For this review, take the finished solid that the model builds, in its own axes (mm). Face numbers are marked on the shaded views. A direction names the side the tool comes from. Coordinates: 2 decimals unless noted, no trailing zeros. Write each loop counter-clockwise with the first axis right and the second up, starting at its lowest first coordinate (ties: lowest second). Pieces come first, ordered by that corner, then holes.
1) We need section C-C on y = 40.5. Write out the cut boundary in (x, z).
2) For the marked faces 5, 6 and 7, list the 3-axis set-ups (+Z, -Z, +X, -X, +Y, -Y) from which the entire face can be reached by the end or side of a thin tool; tool diameter is ignored.
3) To check wall thickness, follow line 1 along Z through (x, y) = (1, 63.5); line 2 along X through (y, z) = (192.5, -11.5); line 3 along X through (y, z) = (135.5, -80.5). State the ranges of each line that lie inside material, in increasing order.
4) We need section B-B on x = 18. Write out the cut boundary in (y, z).
5) We need section D-D on x = 0. Write out the cut boundary in (y, z), then the cut area to 3 significant figures.
6) Mouldability with a two-part tool opening along X and no side actions: class the marked faces 1, 2, 3 and 4 as pulls with the +X half, pulls with the -X half, needs draft (parallel to the pull), parting line crosses it, or undercut.
7) We need section A-A on y = 139. Write out the cut boundary in (x, z), then the cut area to 3 significant figures.
8) Insertion check: P1, Ø9.5, axis at y = 68, z = -114, coming from the +X side; P2, Ø16, axis at y = 39.5, z = -13, coming from the -X side; P3, Ø1.5, axis at x = -34.5, z = -61.5, coming from the -Y side. Each pin has a flat end and moves straight along its axis. Give the tip position at first contact, or say it passes through.
from build123d import *

# Parameters (mm, degrees)
SKETCH1_R                = 23.241
FTA_DEPTH                = 127
SKETCH2_W                = 46.482
SKETCH2_H                = 101.6
FTB_DEPTH                = 32.004
FTC_DEPTH                = 127
SKETCH4_W                = 40.64
SKETCH4_H                = 38.1
FTD1_DEPTH               = 127
SKETCH4_5_W              = 40.64
SKETCH4_5_H              = 38.1
FTD2_DEPTH               = 127
SKETCH5_W                = 25.4
SKETCH5_H                = 48.26
FTE_DEPTH                = 127
FTE_2_DEPTH              = 127
SKETCH6_W                = 40.64
SKETCH6_H                = 48.26
SKETCH6_H_2              = 30.48
FILLER_DEPTH             = 127
BOSS_EXTRUDE1_DEPTH      = 16.002
BOSS_EXTRUDE1_DEPTH_BACK = 16.002
SKETCH8_W                = 46.482
SKETCH8_H                = 101.6
CHAMFER1_SIZE            = 7.62
BOSS_EXTRUDE2_DEPTH      = 32.004
CHAMFER2_SIZE            = 25.4
CHAMFER3_SIZE            = 7.62


with BuildPart() as part:
    # Sketch1 → ftA (new body)
    with BuildSketch(Plane.XY):
        Circle(SKETCH1_R)
    extrude(amount=-FTA_DEPTH)


with BuildPart() as body_2:
    # Sketch2 → ftB (new body)
    with BuildSketch(Plane(origin=(0, 0, -127), x_dir=(-1, 0, 0), z_dir=(0, 0, -1))):
        with Locations((0, 50.8)):
            Rectangle(SKETCH2_W, SKETCH2_H)
    extrude(amount=-FTB_DEPTH)

    # Sketch3 → ftC (add)
    with BuildSketch(Plane(origin=(0, 0, -127), x_dir=(-1, 0, 0), z_dir=(0, 0, -1))):
        Polygon((-23.241, 101.6), (-31.75, 101.6), (-31.75, 132.08), (31.75, 132.08), (31.75, 101.6), (23.241, 101.6), align=None)
    extrude(amount=-FTC_DEPTH)



with BuildPart() as body_3:
    # Sketch4 → ftD1 (new body)
    with BuildSketch(Plane.XY):
        with Locations((52.07, 151.13)):
            Rectangle(SKETCH4_W, SKETCH4_H)
    extrude(amount=-FTD1_DEPTH)

    # Sketch4<5> → ftD2 (add)
    with BuildSketch(Plane.XY):
        with Locations((-52.07, 151.13)):
            Rectangle(SKETCH4_5_W, SKETCH4_5_H)
        with Locations((52.07, 151.13)):
            Rectangle(SKETCH4_5_W, SKETCH4_5_H)
    extrude(amount=-FTD2_DEPTH)


with BuildPart() as ftd2_piece_1:
    # of the separate pieces the step leaves, piece 1, a body of its own (ftd2_pieces)
    add(body_3.part.solids().sort_by_distance((31.75, 132.08, 0))[0])


with BuildPart() as ftd2_piece_2:
    # of the separate pieces the step leaves, piece 2, a body of its own (ftd2_pieces)
    add(body_3.part.solids().sort_by_distance((-31.75, 132.08, 0))[0])


with BuildPart() as body_5:
    # Sketch5 → ftE (new body)
    with BuildSketch(Plane.XY):
        with Locations((-19.05, 194.31)):
            Rectangle(SKETCH5_W, SKETCH5_H)
    extrude(amount=-FTE_DEPTH)


with BuildPart() as body_6:
    # Sketch5 → ftE 2 (new body)
    with BuildSketch(Plane.XY):
        with Locations((19.05, 194.31)):
            Rectangle(SKETCH5_W, SKETCH5_H)
    extrude(amount=-FTE_2_DEPTH)


with BuildPart() as body_2_1:
    add(body_2.part)

    add(ftd2_piece_1.part)  # Filler merges ftD2 piece 1

    add(ftd2_piece_2.part)  # Filler merges ftD2 piece 2

    add(body_5.part)  # Filler merges body 5

    add(body_6.part)  # Filler merges body 6
    # Sketch6 → Filler (add)
    with BuildSketch(Plane.XY):
        with Locations((52.07, 194.31)):
            Rectangle(SKETCH6_W, SKETCH6_H)
        with Locations((-52.07, 194.31)):
            Rectangle(SKETCH6_W, SKETCH6_H)
        with Locations((-52.07, 116.84)):
            Rectangle(SKETCH6_W, SKETCH6_H_2)
        with Locations((52.07, 116.84)):
            Rectangle(SKETCH6_W, SKETCH6_H_2)
    extrude(amount=-FILLER_DEPTH)

    # Combine3: union part
    add(part.part)

    # Sketch8 → Boss-Extrude1 (add, two sides: drawn at the far end of the back side and taken through both)
    with BuildSketch(Plane.XY.offset(-63.5).offset(-BOSS_EXTRUDE1_DEPTH_BACK)):
        with Locations((0, 50.8)):
            Rectangle(SKETCH8_W, SKETCH8_H)
    extrude(amount=BOSS_EXTRUDE1_DEPTH + BOSS_EXTRUDE1_DEPTH_BACK)

    # Chamfer1
    chamfer1_edges = [body_2_1.edges().sort_by_distance(p)[0] for p in [
        (72.39, 101.6, -63.5),
        (0, 101.6, -94.996),
        (-23.241, 101.6, -63.5),
        (0, 101.6, -79.502),
        (23.241, 101.6, -63.5),
        (0, 101.6, -47.498),
        (0, 101.6, 0),
        (-72.39, 101.6, -63.5),
        (23.241, 101.6, -110.998),
        (-23.241, 101.6, -110.998),
    ]]
    chamfer(chamfer1_edges, length=CHAMFER1_SIZE)

    # Sketch9 → Boss-Extrude2 (add)
    with BuildSketch(Plane.XY):
        Polygon((-23.241, 0), (23.241, 0), (23.241, 101.6), (23.241, 109.22), (-23.241, 109.22), (-23.241, 101.6), align=None)
    extrude(amount=-BOSS_EXTRUDE2_DEPTH)

    # Chamfer2
    chamfer2_edges = [body_2_1.edges().sort_by_distance(p)[0] for p in [
        (72.39, 218.44, -63.5),
        (-72.39, 218.44, -63.5),
    ]]
    chamfer(chamfer2_edges, length=CHAMFER2_SIZE)

    # Chamfer3
    chamfer3_edges = [body_2_1.edges().sort_by_distance(p)[0] for p in [
        (0, 101.6, -32.004),
        (-23.241, 101.6, -19.812),
        (23.241, 101.6, -19.812),
    ]]
    chamfer(chamfer3_edges, length=CHAMFER3_SIZE)


solid = body_2_1.part
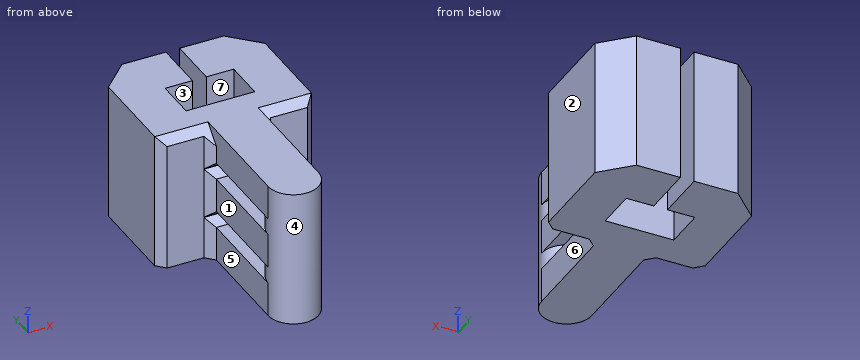
Result:
1. outline: (-23.24, -127) - (23.24, -127) - (23.24, -95) - (-23.24, -95) - close; (-23.24, -79.5) - (23.24, -79.5) - (23.24, -47.5) - (-23.24, -47.5) - close; (-23.24, -32) - (23.24, -32) - (23.24, 0) - (-23.24, 0) - close
2. face 5: +Z, -Z, -X, -Y
2. face 6: +Z, -Z, +X, -Y
2. face 7: +Z, -Z
3. line 1: z = -127 to -95, -79.5 to -47.5, -32 to 0
3. line 2: x = -72.39 to -6.35, 6.35 to 72.39
3. line 3: x = -72.39 to -31.75, 31.75 to 72.39
4. outline: (-14.7, -127) - (132.08, -127) - (132.08, 0) - (-14.7, 0) - close; (170.18, -127) - (218.44, -127) - (218.44, 0) - (170.18, 0) - close; hole (14.7, -95) - (93.98, -95) - (101.6, -87.38) - (101.6, -87.12) - (93.98, -79.5) - (14.7, -79.5) - close; hole (14.7, -47.5) - (93.98, -47.5) - (101.6, -39.88) - (101.6, -39.62) - (93.98, -32) - (14.7, -32) - close
5. outline: (-23.24, -127) - (132.08, -127) - (132.08, 0) - (-23.24, 0) - close; hole (23.24, -95) - (93.98, -95) - (101.6, -87.38) - (101.6, -87.12) - (93.98, -79.5) - (23.24, -79.5) - close; hole (23.24, -47.5) - (93.98, -47.5) - (101.6, -39.88) - (101.6, -39.62) - (93.98, -32) - (23.24, -32) - close
5. area: 17,400 mm2
6. face 1: pulls with the -X half
6. face 2: pulls with the +X half
6. face 3: undercut
6. face 4: parting line crosses it
7. outline: (-72.39, -127) - (-31.75, -127) - (-31.75, 0) - (-72.39, 0) - close; (31.75, -127) - (72.39, -127) - (72.39, 0) - (31.75, 0) - close
7. area: 10,300 mm2
8. P1: stops at x = 23.24
8. P2: stops at x = -23.24
8. P3: stops at y = 101.6
